Source: CAD feature listing. Evaluate the final solid. Frame: model axes, mm. Coordinates: 2 decimals unless noted, no trailing zeros. Write each loop counter-clockwise with the first axis right and the second up, starting at its lowest first coordinate (ties: lowest second). Pieces come first, ordered by that corner, then holes. Notation, with made-up numbers: (40.5, 18) - (93.5, 18) arc R28 ccw to (93.5, 51) - close; hole circle Ø9 at (51.25, -1). An arc over 180 degrees is marked (long way). One line per question, with ' | ' between items.
Autodesk Inventor part; units mm, degrees
ref_plane "YZ Plane" through (0, 0, 0) normal (1, 0, 0) x (0, 1, 0)
ref_plane "XZ Plane" through (0, 0, 0) normal (0, 1, 0) x (-1, 0, 0)
ref_plane "XY Plane" through (0, 0, 0) normal (0, 0, 1) x (1, 0, 0)
sketch "Sketch1" plane through (0, 0, 0) normal (0, 1, 0) x (-1, 0, 0)
  line L0 (-0.5, 0.5) -> (0.5, 0.5)
  line L1 (0.5, 0.5) -> (0.5, -0.5)
  line L2 (0.5, -0.5) -> (-0.5, -0.5)
  line L3 (-0.5, -0.5) -> (-0.5, 0.5)
  line L4 (-0.5, 0.5) -> (0.5, -0.5) construction
  line L5 (0.5, 0.5) -> (-0.5, -0.5) construction
  point P0 (0, 0)
  dimension "d0" = 1
  dimension "d1" = 1
extrude "Extrusion1" add sketch "Sketch1" along normal blind 8
sketch "Sketch2" plane through (0, 0, 0) normal (0, -1, 0) x (1, 0, 0)
  line L0 (-0.32, 0.32) -> (0.32, 0.32)
  line L1 (0.32, 0.32) -> (0.32, -0.32)
  line L2 (0.32, -0.32) -> (-0.32, -0.32)
  line L3 (-0.32, -0.32) -> (-0.32, 0.32)
  line L4 (-0.32, 0.32) -> (0.32, -0.32) construction
  line L5 (0.32, 0.32) -> (-0.32, -0.32) construction
  point P0 (0, 0)
  dimension "d4" = 0.64
  dimension "d5" = 0.64
extrude "Extrusion2" add sketch "Sketch2" along normal blind 14.65
chamfer "Chamfer1" distance 0.155 angle 45 4 edges at (0, -14.65, 0.32) (0.32, -14.65, 0) (0, -14.65, -0.32) (-0.32, -14.65, 0)
sketch "Sketch3" plane through (0, 8, 0) normal (0, 1, 0) x (1, 0, 0)
  line L0 (0.32, 0.32) -> (-0.32, 0.32)
  line L1 (-0.32, 0.32) -> (-0.32, -0.32)
  line L2 (-0.32, -0.32) -> (0.32, -0.32)
  line L3 (0.32, -0.32) -> (0.32, 0.32)
  line L4 (0.32, 0.32) -> (-0.32, -0.32) construction
  line L5 (-0.32, 0.32) -> (0.32, -0.32) construction
  point P0 (0, 0)
  dimension "d11" = 0.64
  dimension "d12" = 0.64
extrude "Extrusion3" cut sketch "Sketch3" against normal blind 6
properties part number "pin" material "Gold"
Item 1: Cut plane C-C on x = 0. Return loops of the section in (y, z) (3 decimals), and give its area (3 significant figures).
Check sheet entries:
outline: (-14.65, -0.165) - (-14.495, -0.32) - (0, -0.32) - (0, -0.5) - (8, -0.5) - (8, -0.32) - (2, -0.32) - (2, 0.32) - (8, 0.32) - (8, 0.5) - (0, 0.5) - (0, 0.32) - (-14.495, 0.32) - (-14.65, 0.165) - close | area: 13.5 mm²
Item 2: Cut plane A-A on z = 0. Return loops of the section in (x, y) (3 decimals).
Check sheet entries:
outline: (-0.5, 0) - (-0.32, 0) - (-0.32, -14.495) - (-0.165, -14.65) - (0.165, -14.65) - (0.32, -14.495) - (0.32, 0) - (0.5, 0) - (0.5, 8) - (0.32, 8) - (0.32, 2) - (-0.32, 2) - (-0.32, 8) - (-0.5, 8) - close
Item 3: Pin query (flat end, axial travel): pin 1 Ø0.5 at (y, z) = (-5, 0) entering from -X. Return the tip coordinate at first contact, or that it passes through.
Check sheet entries:
pin 1: x = -0.32
Item 4: Cut plane D-D on y = -6. Return loops of the section in (x, z).
Check sheet entries:
outline: (-0.32, -0.32) - (0.32, -0.32) - (0.32, 0.32) - (-0.32, 0.32) - close
Item 5: Mould query, pull axis Z, two halves, no side actions, for faces 1 (the face through (0, 4, 0.5)), 2 (the face through (-0.5, 4, 0)), 3 (the face through (0, 4, -0.5)). Classes: pulls with the +Z half, pulls with the -Z half, needs draft (parallel to the pull), parting line crosses it, or undercut.
Check sheet entries:
face 1: pulls with the +Z half | face 2: needs draft | face 3: pulls with the -Z half
Item 6: Cut plane B-B on y = 5. Return loops of the section in (x, z).
Check sheet entries:
outline: (-0.5, -0.5) - (0.5, -0.5) - (0.5, 0.5) - (-0.5, 0.5) - close; hole (-0.32, -0.32) - (0.32, -0.32) - (0.32, 0.32) - (-0.32, 0.32) - close
Item 7: Ray query, line 1 along X through (y, z) = (6.25, -0.25); line 2 along Y through (x, z) = (-0.25, 0.4). Return the intervals inside material, ascending. Write a range as [from, to].
Check sheet entries:
line 1: [-0.5, -0.32], [0.32, 0.5] | line 2: [0, 8]
